Part model, mm, in its own coordinate system. A direction names the side the tool comes from. Give positions to 0.01 mm unless a question says otherwise; leave off trailing zeros. Loops run counter-clockwise (first coordinate to the right, second up) from the corner with the lowest first, then second, coordinate; pieces in that order, holes last. Notation, with made-up numbers: M 50.25,88 L 71.25,88 A15 cw 71.25,112 Z; hole C 38.25,-13 d6. An arc over 180 degrees is marked long. Put each result on its own line as item: value. Start each with the question number.
Autodesk Inventor part; units mm, degrees
ref_plane "YZ Plane" through (0, 0, 0) normal (1, 0, 0) x (0, 1, 0)
ref_plane "XZ Plane" through (0, 0, 0) normal (0, 1, 0) x (-1, 0, 0)
ref_plane "XY Plane" through (0, 0, 0) normal (0, 0, 1) x (1, 0, 0)
sketch "Sketch1" plane through (0, 0, 0) normal (0, 0, 1) x (1, 0, 0)
  circle A0 centre (0, 0) radius 75
  circle A1 centre (0, 0) radius 160
  arc A2 (165, 0) -> (-165, 0) centre (0, 0) ccw
  line L0 (-213, 0) -> (-213, -220)
  line L1 (-213, -220) -> (213, -220)
  line L2 (213, -220) -> (213, 0)
  line L3 (213, 0) -> (165, 0)
  line L4 (-165, 0) -> (-213, 0)
  dimension "inner_diameter" = 150
  dimension "outer_diameter" = 320
  dimension "d37" = 330
  dimension "d38" = 426
  dimension "d39" = 220
  dimension "d40" = 213
  dimension "d41" = 220
extrude "Extrusion1" add sketch "Sketch1" along normal blind 5 contours A1 | L3 L2 L1 L0 L4 A2
sketch "Sketch2" plane through (0, 0, 5) normal (0, 0, 1) x (1, 0, 0)
  circle A0 centre (0, 0) radius 155 construction
  line L0 (0.1758, 0.0573) -> (40.2666, 149.6783) construction
  line L1 (0.1758, 0.0573) -> (-129.7335, 84.4214) construction
  line L2 (0.1758, 0.0573) -> (-120.2034, -97.4238) construction
  line L3 (0.1758, 0.0573) -> (55.6866, -144.5534) construction
  line L4 (0.1758, 0.0573) -> (154.8625, 8.1641) construction
  line L5 (0.1758, 0.0573) -> (0.1758, 154.9999) construction
  dimension "d4" = 310
  dimension "d30" = 360
  dimension "d36" = 15
hole "Hole1" at (40.2666, 149.6783, 5) at (-129.7335, 84.4214, 5) at (-120.2034, -97.4238, 5) at (55.6866, -144.5534, 5) at (154.8625, 8.1641, 5) direction (0, 0, -1) diameter 4.134 depth 8 tip angle 118
sketch "Sketch3" plane through (0, 0, 5) normal (0, 0, 1) x (1, 0, 0)
  circle A0 centre (0, 0) radius 80 construction
  line L0 (0, 0) -> (0, 80) construction
  point P0 (-76.0845, 24.7214)
  point P1 (-76.0845, 24.7214)
  point P2 (-47.0228, -64.7214)
  point P3 (-47.0228, -64.7214)
  point P4 (47.0228, -64.7214)
  point P5 (47.0228, -64.7214)
  point P6 (76.0845, 24.7214)
  point P7 (76.0845, 24.7214)
  dimension "inner_holes_diameter" = 160
  dimension "d34" = 360
hole "Hole2" at (0, 80, 5) at (76.0845, 24.7214, 5) at (47.0228, -64.7214, 5) at (-47.0228, -64.7214, 5) at (-76.0845, 24.7214, 5) direction (0, 0, -1) diameter 4.134 depth 8 tip angle 118
sketch "Sketch5" plane through (0, 0, 5) normal (0, 0, 1) x (1, 0, 0)
  arc A0 (0, -160) -> (80, -138.5641) centre (0, 0) ccw construction
  line L0 (0, 0) -> (0, -160) construction
  line L1 (0, 0) -> (138.5641, -80) construction
  line L2 (0, 0) -> (80, -138.5641) construction
  arc A1 (138.5641, -80) -> (0, -160) centre (0, 0) ccw construction
  arc A2 (84.1622, -136.0762) -> (136.0762, -84.1622) centre (0, 0) ccw
  line L3 (82.4621, -142.8286) -> (111.1399, -192.5)
  line L4 (142.8286, -82.4621) -> (185.5, -107.0985)
  arc A3 (142.8286, -82.4621) -> (136.0762, -84.1622) centre (140.3286, -86.7922) ccw
  arc A4 (84.1622, -136.0762) -> (82.4621, -142.8286) centre (86.7922, -140.3286) ccw
  line L5 (188, -190) -> (188, -111.4286)
  line L6 (183, -195) -> (115.4701, -195)
  arc A5 (111.1399, -192.5) -> (115.4701, -195) centre (115.4701, -190) ccw
  arc A6 (188, -111.4286) -> (185.5, -107.0985) centre (183, -111.4286) ccw
  arc A7 (183, -195) -> (188, -190) centre (183, -190) ccw
  line L7 (213, -220) -> (213, 0)
  line L8 (-213, -220) -> (213, -220)
  point P0 (188, -108.5419)
  point P1 (112.5833, -195)
  point P2 (188, -195)
  dimension "d50" = 320
  dimension "d52" = 30
  dimension "d53" = 30
  dimension "d54" = 5
  dimension "d68" = 5
  dimension "d69" = 5
  dimension "d70" = 25
  dimension "d71" = 25
extrude "Extrusion3" cut sketch "Sketch5" against normal blind 3
sketch "Sketch6" plane through (0, 0, 5) normal (0, 0, 1) x (1, 0, 0)
  arc A0 (142.8286, -82.4621) -> (136.0762, -84.1622) centre (140.3286, -86.7922) ccw
  arc A1 (84.1622, -136.0762) -> (136.0762, -84.1622) centre (0, 0) ccw
  arc A2 (84.1622, -136.0762) -> (82.4621, -142.8286) centre (86.7922, -140.3286) ccw
  line L0 (111.1399, -192.5) -> (82.4621, -142.8286)
  line L1 (142.8286, -82.4621) -> (185.5, -107.0985)
  circle A3 centre (0, 0) radius 170 construction
  circle A4 centre (0, 0) radius 187.5 construction
  line L2 (0, 0) -> (0, -170) construction
  line L3 (0, 0) -> (79.2409, -169.9327) construction
  line L4 (0, 0) -> (169.9327, -79.2409) construction
  line L5 (183, -195) -> (115.4701, -195)
  line L6 (188, -111.4286) -> (188, -190)
  arc A5 (111.1399, -192.5) -> (115.4701, -195) centre (115.4701, -190) ccw
  arc A6 (183, -195) -> (188, -190) centre (183, -190) ccw
  arc A7 (188, -111.4286) -> (185.5, -107.0985) centre (183, -111.4286) ccw
  point P0 (71.8451, -154.0723)
  point P1 (154.0723, -71.8451)
  dimension "d57" = 340
  dimension "d58" = 375
  dimension "d59" = 25
  dimension "d60" = 40
hole "Hole3" at (71.8451, -154.0723, 5) at (79.2409, -169.9327, 5) at (169.9327, -79.2409, 5) at (154.0723, -71.8451, 5) direction (0, 0, -1) diameter 4.134 end through all
equation "\"inner_diameter\" = id"
equation "\"outer_diameter\" = od"
equation "\"d50\" = od"
equation "\"id\" = 150"
equation "\"od\" = 320"
properties part number "bakplate"
1) Mould opens along X. For faces 3 (the flat face through (96.6, -167.32, 3.52)), 4 (the flat face through (44, -68, 0)), 5 (the cylindrical face through (-3.63, 164.96, 2.46)), 6 (the flat face through (146, -150, 2)) say: +X half, -X half, draft (parallel to the pull), parting line (faces both ways), or undercut.
2) Band-saw the part on A-A on x = 14. Give the cut face in (y, z).
3) Wall check: L1, parallel to Y at x = 1, z = 0.9; L2, parallel to X at y = -152.5, z = 3.8; L3, parallel to Y at x = 17.5, z = 1.2. Give the ranges that are in metal, low to high.
4) Band-saw the part on B-B on z = 0.9. State how many separate pieces and enclosed holes the cut face has, then the cut area to 3 significant figures.
5) Which spindle directions (+Z, -Z, +X, -X, +Y, -Y) get a long thin tool onto all of the face, cutting with end or side? Do faces 1 (the flat face through (-50, -68, 5)), 2 (the flat face through (163.87, -94.61, 3.52)). Say none if no direction does.
6) Pin check, flat tips, straight feed: pin 1 Ø3.5 at (x, y) = (-120.2, -97.42) entering from +Z; pin 2 Ø1.5 at (x, z) = (-191.5, 3.5) entering from +Y; pin 3 Ø1.5 at (y, z) = (13, 2) entering from +X. Stop position of each tip, or through.
7) Band-saw the part on C-C on x = 97.5. Give the cut face in (y, z) (3 decimals), then the cut area to 3 significant figures.
8) Band-saw the part on D-D on y = 133. Give the cut face in (x, z), then the cut area to 3 significant figures.
Evaluation:
1. face 3: undercut
1. face 4: draft
1. face 5: parting line
1. face 6: undercut
2. outline: M -220,0 L -73.68,0 L -73.68,5 L -220,5 Z; M 73.68,0 L 164.4,0 L 164.4,5 L 73.68,5 Z
3. L1: -220 to -74.99, 74.99 to 78.19, 81.81 to 165
3. L2: -213 to 70.5, 73.19 to 88.05, 188 to 213
3. L3: -220 to -72.93, 72.93 to 164.07
4. separate pieces: 1
4. enclosed holes: 15
4. area: 119,000 mm2
5. face 1: +Z, +X, -X, +Y, -Y
5. face 2: +Z
6. pin 1: through
6. pin 2: y = 0
6. pin 3: x = 164.54
7. outline: M -220,0 L 133.112,0 L 133.112,5 L -126.861,5 L -126.861,2 L -168.875,2 L -168.875,5 L -220,5 Z
7. area: 1,640 mm2
8. outline: M -97.65,0 L 97.65,0 L 97.65,5 L -97.65,5 Z
8. area: 977 mm2
